Part model, mm, in its own coordinate system. Give positions to 0.01 mm unless a question says otherwise; leave off trailing zeros. Write each loop counter-clockwise with the first axis right and the second up, starting at its lowest first coordinate (ties: lowest second). Pieces come first, ordered by that corner, then holes. Notation, with made-up numbers: M -23.75,-36 L -19.75,-36 A23 cw -19.75,-2 Z; hole C 52.25,82 d8. An arc over 180 degrees is marked long. Use CSV: the item, a comma, the result in double quotes. Start each with the question number.
Item 1: Cut at A-A (x = 30). List the corners of the cut face in (y, z), then the cut area to 3 significant figures.
Item 2: Drill centre lines: line 1 (Y direction, x = 184.5, z = 7.5); line 2 (Y direction, x = 0, z = 4.5); line 3 (Y direction, x = 166.5, z = 8). Where is each one in solid material? Low to high. Write a range as [from, to].
Item 3: Pin check, flat tips, straight feed: pin 1 (5 mm diameter, centred on x = 0.5, y = -1.5, fed in from +Z); pin 2 (4 mm diameter, centred on y = -6, z = 4, fed in from -X); pin 3 (2 mm diameter, centred on y = -3, z = 6.5, fed in from +X). Stop position of each tip, or through.
Item 4: Cut at B-B (z = 5.25). Count the separate pieces of the cut face and the enclosed holes in it, then the cut area to 3 significant figures.
Item 5: Cut at C-C (x = 67). List the corners of the cut face in (y, z), then the cut area to 3 significant figures.
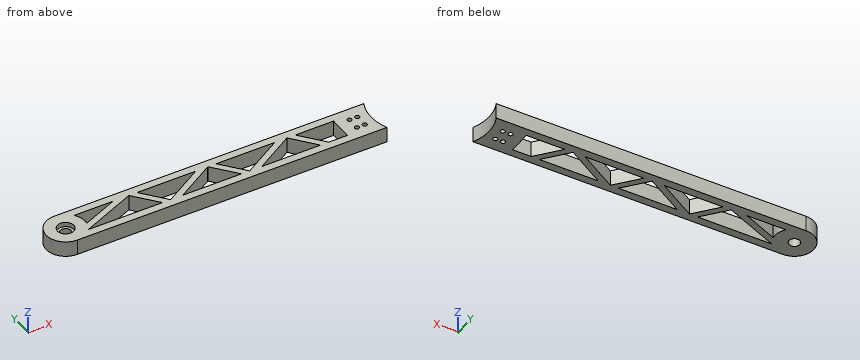
from build123d import *

# Parameters (mm, degrees)
EXTRUDE_1_DEPTH          = 10
CUT_EXTRUDE_1_DEPTH      = 252.652538235
CUT_EXTRUDE_1_DEPTH_BACK = 252.652538235
SKETCH_7_R               = 3.5
CUT_EXTRUDE_5_DEPTH      = 252.652538235
SKETCH_8_R               = 5
CUT_EXTRUDE_6_DEPTH      = 3
SKETCH_9_R               = 3
CUT_EXTRUDE_7_DEPTH      = 252.652538235
SKETCH_10_R              = 5.25
CUT_EXTRUDE_8_DEPTH      = 3
CUT_EXTRUDE_START        = -10
SKETCH_11_R              = 27
CUT_EXTRUDE_9_DEPTH      = 10
SKETCH_12_R              = 30
CUT_EXTRUDE_10_DEPTH     = 10
SKETCH_14_R              = 1.45
CUT_EXTRUDE_12_DEPTH     = 300


with BuildPart() as part:
    # 草图1 → 凸台-拉伸1 (new body)
    with BuildSketch(Plane.XY):
        with BuildLine():
            Line((0, 12.5), (199.067804112, 12.5))
            ThreePointArc((199.067804112, 12.5), (250, 0), (199.067804112, -12.5))
            Line((199.067804112, -12.5), (0, -12.5))
            ThreePointArc((0, -12.5), (-12.5, 0), (0, 12.5))
        make_face()
    extrude(amount=EXTRUDE_1_DEPTH)

    # 草图3 → 切除-拉伸1 (cut, two sides: drawn at the far end of the back side and taken through both)
    with BuildSketch(Plane.XY.offset(10).offset(-CUT_EXTRUDE_1_DEPTH_BACK)):
        Polygon((176.376805713, 7.5), (151.73545401, 7.5), (164.376805713, -7.5), (176.376805713, -7.5), align=None)
        Polygon((159.145761472, -7.5), (146.504409769, 7.5), (146.399203355, 7.5), (121.399203355, -7.5), align=None)
        Polygon((113.624600829, -7.5), (138.624600829, 7.5), (100.983249125, 7.5), align=None)
        Polygon((70.646998471, -7.5), (108.393556588, -7.5), (95.752204884, 7.5), (95.646998471, 7.5), align=None)
        Polygon((50.231044241, 7.5), (62.872395944, -7.5), (87.872395944, 7.5), align=None)
        Polygon((10, -7.5), (57.641351703, -7.5), (45, 7.5), align=None)
        with BuildLine():
            Line((34.845635859, 7.5), (10, 7.5))
            ThreePointArc((10, 7.5), (12.156331085, 2.910947362), (12.312475569, -2.157068696))
            Line((12.312475569, -2.157068696), (34.845635859, 7.5))
        make_face()
    extrude(amount=CUT_EXTRUDE_1_DEPTH + CUT_EXTRUDE_1_DEPTH_BACK, mode=Mode.SUBTRACT)

    # 草图7 → 切除-拉伸5 (cut, through all)
    with BuildSketch(Plane(origin=(0, 0, 0), x_dir=(-1, 0, 0), z_dir=(0, 0, -1))):
        Circle(SKETCH_7_R)
    extrude(amount=-CUT_EXTRUDE_5_DEPTH, mode=Mode.SUBTRACT)

    # 草图8 → 切除-拉伸6 (cut)
    with BuildSketch(Plane(origin=(0, 0, 0), x_dir=(-1, 0, 0), z_dir=(0, 0, -1))):
        with Locations((-223, 0)):
            Circle(SKETCH_8_R)
    extrude(amount=-CUT_EXTRUDE_6_DEPTH, mode=Mode.SUBTRACT)

    # 草图9 → 切除-拉伸7 (cut, through all)
    with BuildSketch(Plane(origin=(0, 0, 0), x_dir=(-1, 0, 0), z_dir=(0, 0, -1))):
        with Locations((-223, 0)):
            Circle(SKETCH_9_R)
    extrude(amount=-CUT_EXTRUDE_7_DEPTH, mode=Mode.SUBTRACT)

    # 草图10 → 切除-拉伸8 (cut)
    with BuildSketch(Plane.XY.offset(10)):
        Circle(SKETCH_10_R)
    extrude(amount=-CUT_EXTRUDE_8_DEPTH, mode=Mode.SUBTRACT)

    # 草图11 → 切除-拉伸9 (cut)
    with BuildSketch(Plane.XY.offset(10).offset(CUT_EXTRUDE_START)):
        with Locations((223, 0)):
            Circle(SKETCH_11_R)
    extrude(amount=CUT_EXTRUDE_9_DEPTH, mode=Mode.SUBTRACT)

    # 草图12 → 切除-拉伸10 (cut)
    with BuildSketch(Plane.XY.offset(10)):
        with Locations((226, 0)):
            Circle(SKETCH_12_R)
    extrude(amount=-CUT_EXTRUDE_10_DEPTH, mode=Mode.SUBTRACT)

    # 草图14 → 切除-拉伸12 (cut)
    with BuildSketch(Plane.XY.offset(10)):
        with Locations((184.5, 4)):
            Circle(SKETCH_14_R)
        with Locations((189.5, 4)):
            Circle(SKETCH_14_R)
        with Locations((189.5, -4)):
            Circle(SKETCH_14_R)
        with Locations((184.5, -4)):
            Circle(SKETCH_14_R)
    extrude(amount=-CUT_EXTRUDE_12_DEPTH, mode=Mode.SUBTRACT)


solid = part.part
Worked answers:
1,outline,"M -12.5,0 L -7.5,0 L -7.5,10 L -12.5,10 Z; M 1.07,0 L 5.42,0 L 5.42,10 L 1.07,10 Z; M 7.5,0 L 12.5,0 L 12.5,10 L 7.5,10 Z"
1,area,"144 mm^2"
2,line 1,"y = [-12.5, -5.45], [-2.55, 2.55], [5.45, 12.5]"
2,line 2,"y = [-12.5, -3.5], [3.5, 12.5]"
2,line 3,"y = [-12.5, -7.5], [7.5, 12.5]"
3,pin 1,"stops at z = 7"
3,pin 2,"stops at x = -11.84"
3,pin 3,"stops at x = 196.27"
4,separate pieces,"1"
4,enclosed holes,"12"
4,area,"3,230 mm^2"
5,outline,"M -12.5,0 L -5.02,0 L -5.02,10 L -12.5,10 Z; M 7.5,0 L 12.5,0 L 12.5,10 L 7.5,10 Z"
5,area,"125 mm^2"
